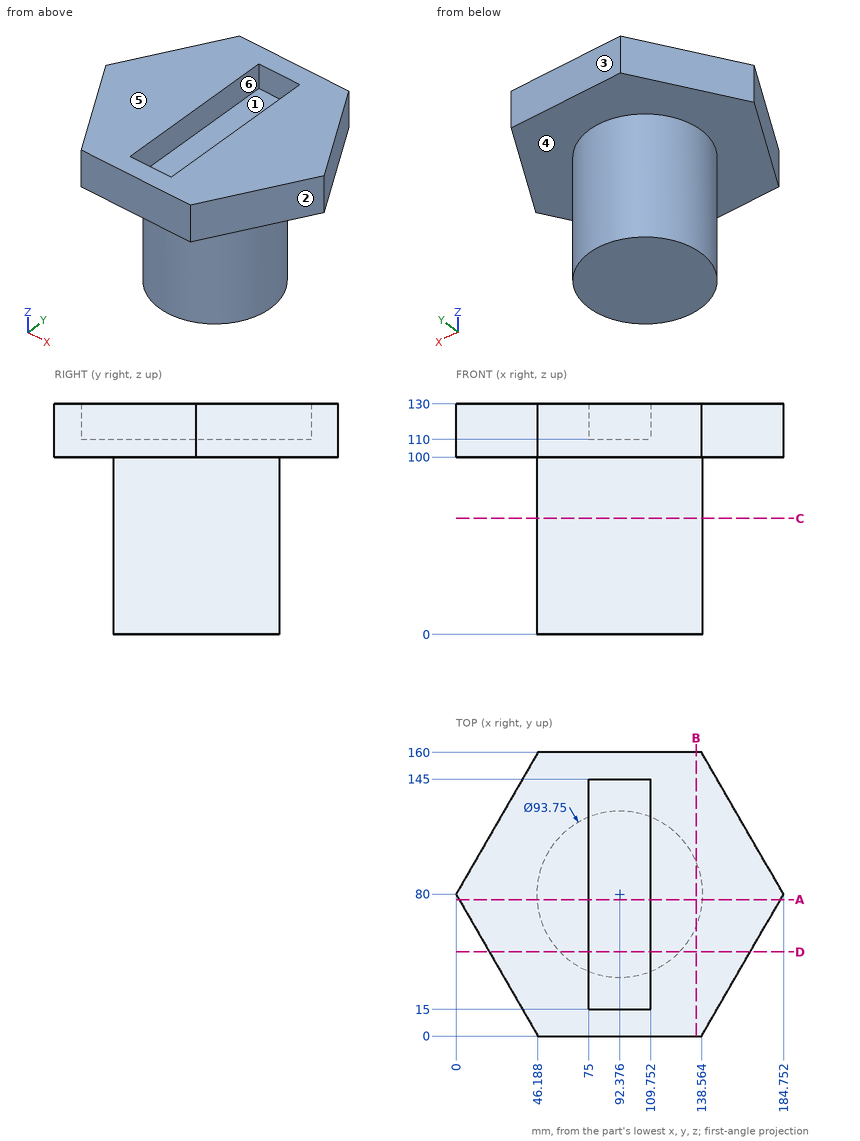
Job drawing, mm, ordinate dimensions from the low corner. One solid piece. A direction names the side the tool comes from. Round coordinates to 2 decimals unless told otherwise and drop trailing zeros. Order: outer loops, then holes, each group sorted by start corner. A loop starts at its lowest first (then second) coordinate and runs counter-clockwise, first axis right, second up. Notation, with made-up numbers: (-12, 88) -> (35, 88) arc R12 ccw to (35, 94) -> close; hole circle Ø1 at (32, 6). An arc over 180 degrees is marked (long way). Write item = value, one per line.
(1) Cut at C-C (z = 65.5). Write the cut outline in (x, y) (3 decimals).
Answers follow:
outline = circle Ø93.75 at (92.376, 80)
(2) 3-axis set-ups, long thin cutter, end or side, ignore diameter. For the marked faces 4, 5 and 6: which of +Z, -Z, +X, -X, +Y, -Y reach the whole face in a straight line?
Answers follow:
face_4 = -Z
face_5 = +Z, +X, -X, +Y, -Y
face_6 = +Z
(3) Cut at A-A (y = 77). Write the cut outline in (x, z) (3 decimals), plus the area to 3 significant figures.
Answers follow:
outline = (1.732, 100) -> (45.597, 100) -> (45.597, 0) -> (139.155, 0) -> (139.155, 100) -> (183.02, 100) -> (183.02, 130) -> (109.752, 130) -> (109.752, 110) -> (75, 110) -> (75, 130) -> (1.732, 130) -> close
area = 14,100 mm²
(4) Flat gauge pins, fed straight in: P1, Ø10, axis at x = 49.5, z = 27, coming from the -Y side; P2, Ø22, axis at y = 65, z = 117, coming from the +X side; P3, Ø8, axis at x = 74.5, z = 30.5, coming from the -Y side. Where does each tip first touch, or does it go through?
Answers follow:
P1 = 52.38
P2 = 182.44
P3 = 35.23
(5) Drill centre lines: L1, parallel to Y at x = 104.5, z = 117; L2, parallel to Z at x = 124.5, y = 125; L3, parallel to Z at x = 102.5, y = 77. Where is each one in solid material? Low to high.
Answers follow:
L1 = 0 to 15, 145 to 160
L2 = 100 to 130
L3 = 0 to 110
(6) Cut at D-D (y = 47.5). Write the cut outline in (x, z) (3 decimals), plus the area to 3 significant figures.
Answers follow:
outline = (18.764, 100) -> (58.597, 100) -> (58.597, 0) -> (126.155, 0) -> (126.155, 100) -> (165.988, 100) -> (165.988, 130) -> (109.752, 130) -> (109.752, 110) -> (75, 110) -> (75, 130) -> (18.764, 130) -> close
area = 10,500 mm²
(7) Cut at B-B (x = 135.5). Write the cut outline in (y, z), plus the area to 3 significant figures.
Answers follow:
outline = (0, 100) -> (61.63, 100) -> (61.63, 0) -> (98.37, 0) -> (98.37, 100) -> (160, 100) -> (160, 130) -> (0, 130) -> close
area = 8,470 mm²
(8) Pull direction X, two halves, no side cores. Call the marked faces 1, 2 and 3: +X half, -X half, draft (parallel to the pull), parting line (faces both ways), or undercut.
Answers follow:
face_1 = undercut
face_2 = +X half
face_3 = draft
